Verification items for this drawing (mm, ordinates from the low corner). A direction names the side the tool comes from. Round coordinates to 2 decimals unless told otherwise and drop trailing zeros. Order: outer loops, then holes, each group sorted by start corner. A loop starts at its lowest first (then second) coordinate and runs counter-clockwise, first axis right, second up. Notation, with made-up numbers: (-24, 56) -> (29, 56) arc R19 cw to (29, 76) -> close; hole circle Ø1 at (50, -33.75). An arc over 180 degrees is marked (long way). Use a Markdown table: item, result. Add a question column.
Item 1: Set-up check for the marked faces 5 and 6: record each of +Z, -Z, +X, -X, +Y, -Y from which the full face is reachable in a straight line by a thin tool's end or side.
Item 2: Sectioned sample at A-A, the plane z = 9.75. Record the cut outline in (x, y) (1 decimal).
Item 3: Mould release check, pull along X, two halves, no side actions. Record for the marked faces 1, 2, 3 and 4: pulls with the +X half, pulls with the -X half, needs draft (parallel to the pull), parting line crosses it, or undercut.
Item 4: Sectioned sample at B-B, the plane z = 1. Record the cut outline in (x, y).
Item 5: Material ranges on probe 1 along X at (y, z) = (3, 8.25); probe 2 along Z at (x, y) = (1.5, 5); probe 3 along Y at (x, z) = (3.6, 10.5) (1 decimal), recorded low to high. Write a range as [from, to].
Item 6: Gauge pin test, flat ends, axial feed: pin 1 Ø3 at (y, z) = (5, 2.5) entering from +X (1 decimal); pin 2 Ø3 at (x, z) = (1.5, 2.5) entering from -Y; pin 3 Ø2.5 at (x, y) = (3.5, 2) entering from -Z. Record the tip position at first contact, or that the pin passes through.
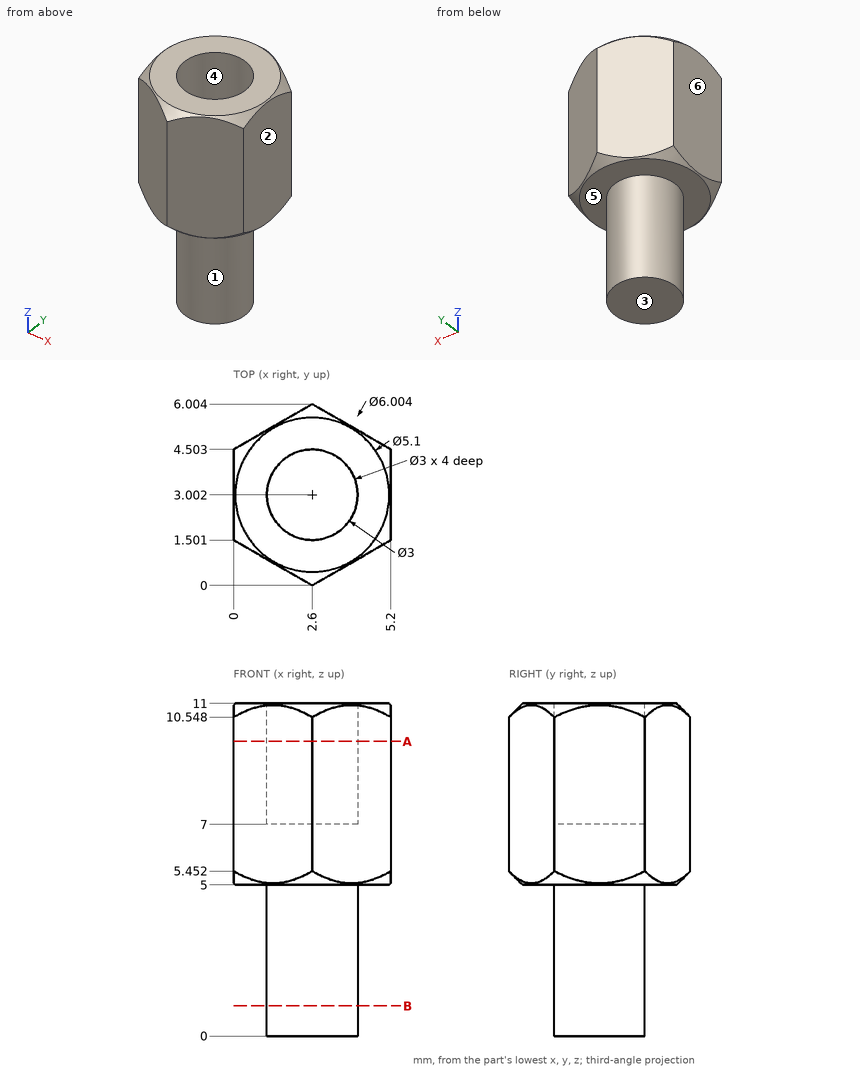
Found:
| question | item | result |
|---|---|---|
| 1 | face 5 | -Z |
| 1 | face 6 | +Z, -Z, -X, +Y, -Y |
| 2 | outline | (0, 1.5) -> (2.6, 0) -> (5.2, 1.5) -> (5.2, 4.5) -> (2.6, 6) -> (0, 4.5) -> close; hole circle Ø3 at (2.6, 3) |
| 3 | face 1 | parting line crosses it |
| 3 | face 2 | pulls with the +X half |
| 3 | face 3 | needs draft |
| 3 | face 4 | undercut |
| 4 | outline | circle Ø3 at (2.6, 3) |
| 5 | probe 1 | x = [0, 1.1], [4.1, 5.2] |
| 5 | probe 2 | z = [5, 11] |
| 5 | probe 3 | y = [0.6, 1.9], [4.1, 5.4] |
| 6 | pin 1 | stops at x = 4 |
| 6 | pin 2 | stops at y = 1.5 |
| 6 | pin 3 | stops at z = 0 |
